Read the model definition and answer for the solid it produces. Units are mm, in the model's axes. Coordinates: 2 decimals unless noted, no trailing zeros. Write each loop counter-clockwise with the first axis right and the second up, starting at its lowest first coordinate (ties: lowest second). Pieces come first, ordered by that corner, then holes.
from build123d import *

# Parameters (mm, degrees)
SKETCH1_W                             = 69.85
SKETCH1_H                             = 25.4
EXTRUDE1_DEPTH                        = 1.5748
F_1_8_0_125_DIAMETER_HOLE1_AT_2_COUNT = 2
F_1_8_0_125_DIAMETER_HOLE1_AT_2_PITCH = 57.13222


with BuildPart() as part:
    # Sketch1 → Extrude1 (new body)
    with BuildSketch(Plane.XY):
        Rectangle(SKETCH1_W, SKETCH1_H)
    extrude(amount=EXTRUDE1_DEPTH)

    # Sketch3 → 1/8 (0.125) Diameter Hole1 (revolve, cut)
    with BuildSketch(Plane(origin=(-25.38222, 9.525, 1.5748), x_dir=(0, -1, 0), z_dir=(1, 0, 0))):
        Polygon((0, 0), (0, 16.955866233), (1.5875, 16.002), (1.5875, 0), align=None)
    f_1_8_0_125_diameter_hole1 = revolve(axis=Axis((-25.38222, 9.525, 7.9248), (0, 0, -1)), mode=Mode.SUBTRACT)

    # 1/8 (0.125) Diameter Hole1 at 2: 1/8 (0.125) Diameter Hole1 ×2
    with Locations(*[(i * F_1_8_0_125_DIAMETER_HOLE1_AT_2_PITCH, 0, 0) for i in range(1, F_1_8_0_125_DIAMETER_HOLE1_AT_2_COUNT)]):
        add(f_1_8_0_125_diameter_hole1, mode=Mode.SUBTRACT)

    # Mirror1: 1/8 (0.125) Diameter Hole1 across plane
    add(f_1_8_0_125_diameter_hole1.mirror(Plane.ZX), mode=Mode.SUBTRACT)

    # Mirror1 copy 1 sketch → Mirror1 copy 1 (revolve, cut)
    with BuildSketch(Plane(origin=(31.75, -9.525, 1.5748), x_dir=(0, 1, 0), z_dir=(1, 0, 0))):
        Polygon((0, 0), (0, -16.955866233), (1.5875, -16.002), (1.5875, 0), align=None)
    revolve(axis=Axis((31.75, -9.525, 7.9248), (0, 0, 1)), mode=Mode.SUBTRACT)


solid = part.part
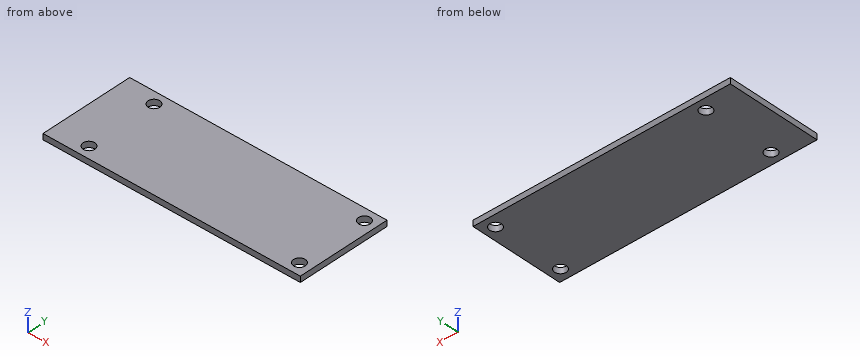
Item 1: The part is cut by section A-A (x = 31.75). Give the vertices of the cut face in (y, z), and give its area (3 significant figures).
Item 2: Find the intervals of material crossed by probe 1 along X at (y, z) = (-10.75, 0.55) (1 decimal), in increasing order.
Item 3: The part is cut by section B-B (z = 1.2). State how many separate pieces and enclosed holes the cut face has, and give its area (3 significant figures).
Answer:
1. outline: (-12.7, 0) - (-11.11, 0) - (-11.11, 1.57) - (-12.7, 1.57) - close; (-7.94, 0) - (7.94, 0) - (7.94, 1.57) - (-7.94, 1.57) - close; (11.11, 0) - (12.7, 0) - (12.7, 1.57) - (11.11, 1.57) - close
1. area: 30.0 mm2
2. probe 1: x = -34.9 to -26.4, -24.4 to 30.7, 32.8 to 34.9
3. separate pieces: 1
3. enclosed holes: 4
3. area: 1,740 mm2
